```python
from build123d import *

# Parameters (mm, degrees)
BOSS_EXTRUDE1_DEPTH            = 9
CBORE_FOR_M5_SHCS1_D           = 5.5
CBORE_FOR_M5_SHCS1_CBORE_D     = 10
CBORE_FOR_M5_SHCS1_CBORE_DEPTH = 5
F_1_0MM_DOWEL_HOLE1_D          = 16.1
F_1_0MM_DOWEL_HOLE1_DEPTH      = 5.3
F_1_0MM_DOWEL_HOLE3_D          = 12
SKETCH14_R                     = 3.2
CUT_EXTRUDE1_DEPTH             = 68.490740106
CHAMFER1_SIZE                  = 3


with BuildPart() as part:
    # Sketch1 → Boss-Extrude1 (new body)
    with BuildSketch(Plane(origin=(0, 0, 0), x_dir=(1, 0, 0), z_dir=(0, 1, 0))):
        Polygon((2, -45), (35, -45), (35, 45), (-25, 45), (-25, -57), (2, -57), align=None)
    extrude(amount=BOSS_EXTRUDE1_DEPTH)

    # CBORE for M5 SHCS1 (through all)
    with Locations(Plane(origin=(0, 9, 0), x_dir=(1, 0, 0), z_dir=(0, 1, 0))):
        with Locations((27.5, 37.5), (27.5, -37.5), (-11.5, 11), (-11.5, -49.5)):
            CounterBoreHole(CBORE_FOR_M5_SHCS1_D / 2, CBORE_FOR_M5_SHCS1_CBORE_D / 2, CBORE_FOR_M5_SHCS1_CBORE_DEPTH)

    # Ø1.0mm Dowel Hole1
    with Locations(Plane(origin=(0, 9, 0), x_dir=(1, 0, 0), z_dir=(0, 1, 0))):
        with Locations((0, 30)):
            Hole(F_1_0MM_DOWEL_HOLE1_D / 2, depth=F_1_0MM_DOWEL_HOLE1_DEPTH)

    # Ø1.0mm Dowel Hole3 (through all)
    with Locations(Plane(origin=(0, 3.7, 0), x_dir=(1, 0, 0), z_dir=(0, 1, 0))):
        with Locations((0, 30)):
            Hole(F_1_0MM_DOWEL_HOLE3_D / 2)

    # Sketch14 → Cut-Extrude1 (cut, through all)
    with BuildSketch(Plane(origin=(0, 9, 0), x_dir=(1, 0, 0), z_dir=(0, 1, 0))):
        with Locations(Location((12, -28.35, 0), (0, 0, 270))):
            Circle(SKETCH14_R)
        with Locations(Location((-12, -28.35, 0), (0, 0, 270))):
            Circle(SKETCH14_R)
    extrude(amount=-CUT_EXTRUDE1_DEPTH, mode=Mode.SUBTRACT)

    # Chamfer1
    chamfer1_edges = [part.edges().sort_by_distance(p)[0] for p in [
        (35, 4.5, 45),
        (2, 4.5, 45),
        (2, 4.5, 57),
        (-25, 4.5, 57),
        (-25, 4.5, -45),
        (35, 4.5, -45),
    ]]
    chamfer(chamfer1_edges, length=CHAMFER1_SIZE)


solid = part.part
```
Source: CAD feature listing. Evaluate the final solid. Frame: model axes, mm. A direction names the side the tool comes from. Round coordinates to 2 decimals unless told otherwise and drop trailing zeros. Order: outer loops, then holes, each group sorted by start corner. A loop starts at its lowest first (then second) coordinate and runs counter-clockwise, first axis right, second up. Notation, with made-up numbers: (69, -12.5) -> (110, -12.5) arc R13 cw to (110, 2.5) -> close; hole circle Ø11 at (79, -27.5). An arc over 180 degrees is marked (long way). One line per item, written item: value. Start each with the question number.
Q1. Pin query (flat end, axial travel): pin 1 (1 mm diameter, centred on x = 27.5, y = 3, fed in from +Z); pin 2 (5 mm diameter, centred on x = -1.5, z = -26.5, fed in from +Y); pin 3 (9.5 mm diameter, centred on x = 0, z = -30, fed in from +Y); pin 4 (3 mm diameter, centred on x = 26, z = -35.5, fed in from +Y). Return the tip coordinate at first contact, or that it passes through.
Q2. Section query D-D (z = -30). Return the cut outline in (x, y), plus the area to 3 significant figures.
Q3. Section query C-C (y = 5.5). Return the cut outline in (x, z), plus the area to 3 significant figures.
Q4. Draft query along Z for faces 1 (the cylindrical face through (23.815, 6.535, -40.879)), 2 (the flat face through (5, 0, 5)), 3 (the flat face through (3, 4, 47)). Return one class per face: pulls with the +Z half, pulls with the -Z half, needs draft (parallel to the pull), parting line crosses it, or undercut.
Q5. Section query A-A (z = 28.35). Return the cut outline in (x, y), plus the area to 3 significant figures.
Q6. Section query B-B (x = 0). Return the cut outline in (y, z).
Q7. Material intervals for probe 1 along X at (y, z) = (1.8, -11); probe 2 along X at (y, z) = (4.75, -33); probe 3 along Z at (x, y) = (-11.5, 2.4), sorted ascending.
Q8. Access query for faces 4 (the flat face through (18, 4, 45)), 5 (the cylindrical face through (1.745, 6.313, -22.141)), 6 (the cylindrical face through (1.301, 1.824, -24.143)). Directions: +Z, -Z, +X, -X, +Y, -Y. A direction counts if a zero-diameter tool reaches every point of the face in a straight line with its end or side. Return the directions, or none.
Findings below:
1. pin 1: z = 45
1. pin 2: y = 3.7
1. pin 3: through
1. pin 4: y = 4
2. outline: (-25, 0) -> (-6, 0) -> (-6, 3.7) -> (-8.05, 3.7) -> (-8.05, 9) -> (-25, 9) -> close; (6, 0) -> (35, 0) -> (35, 9) -> (8.05, 9) -> (8.05, 3.7) -> (6, 3.7) -> close
2. area: 410 mm²
3. outline: (-25, -42) -> (-22, -45) -> (32, -45) -> (35, -42) -> (35, 42) -> (32, 45) -> (5, 45) -> (2, 48) -> (2, 54) -> (-1, 57) -> (-22, 57) -> (-25, 54) -> close; hole circle Ø10 at (-11.5, -11); hole circle Ø10 at (-11.5, 49.5); hole circle Ø6.4 at (-12, 28.35); hole circle Ø16.1 at (0, -30); hole circle Ø6.4 at (12, 28.35); hole circle Ø10 at (27.5, -37.5); hole circle Ø10 at (27.5, 37.5)
3. area: 5,120 mm²
4. face 1: undercut
4. face 2: needs draft
4. face 3: pulls with the +Z half
5. outline: (-25, 0) -> (-15.2, 0) -> (-15.2, 9) -> (-25, 9) -> close; (-8.8, 0) -> (8.8, 0) -> (8.8, 9) -> (-8.8, 9) -> close; (15.2, 0) -> (35, 0) -> (35, 9) -> (15.2, 9) -> close
5. area: 425 mm²
6. outline: (0, -45) -> (9, -45) -> (9, -38.05) -> (3.7, -38.05) -> (3.7, -36) -> (0, -36) -> close; (0, -24) -> (3.7, -24) -> (3.7, -21.95) -> (9, -21.95) -> (9, 56) -> (0, 56) -> close
7. probe 1: -25 to -14.25, -8.75 to 35
7. probe 2: -25 to -7.47, 7.47 to 25.32, 29.68 to 35
7. probe 3: -45 to -13.75, -8.25 to 25.19, 31.51 to 46.75, 52.25 to 57
8. face 4: +Z, +X, +Y, -Y
8. face 5: +Y
8. face 6: +Y, -Y
